The figure shows three views and two pictorial views of one solid part (mm, origin at its lowest corner). Answer the questions. A direction names the side the tool comes from. Coordinates: 2 decimals unless noted, no trailing zeros. Write each loop counter-clockwise with the first axis right and the second up, starting at its lowest first coordinate (ties: lowest second). Pieces come first, ordered by that corner, then holes.
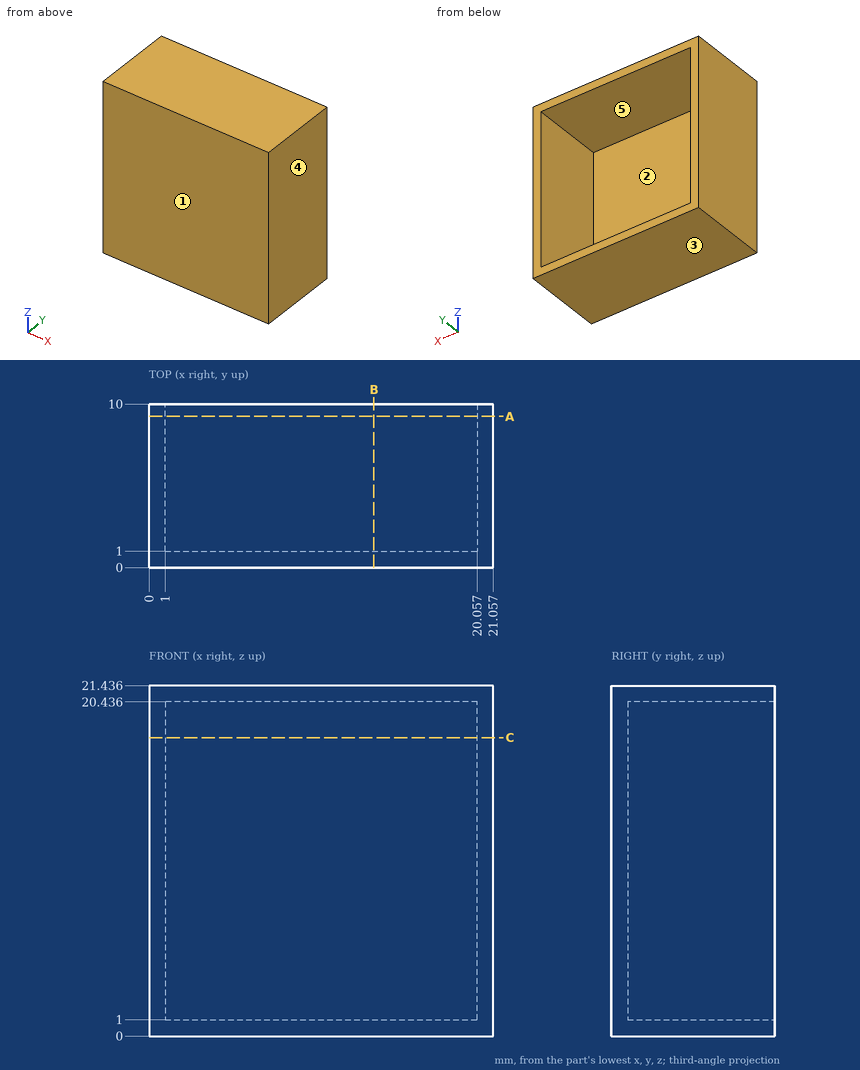
1. Section A-A on y = 9.25 is taken. Give the vertices of the cut face in (x, z) (1 decimal).
Results found:
outline: (0, 0) - (21.1, 0) - (21.1, 21.4) - (0, 21.4) - close; hole (1, 1) - (20.1, 1) - (20.1, 20.4) - (1, 20.4) - close
2. Find the intervals of material crossed by L1, parallel to X at y = 4, z = 1.25; L2, parallel to Z at x = 14, y = 7 (1 decimal); L3, parallel to Y at x = 10.5, z = 5.25, in increasing order.
Results found:
L1: x = 0 to 1, 20.06 to 21.06
L2: z = 0 to 1, 20.4 to 21.4
L3: y = 0 to 1
3. Section C-C on z = 18.25 is taken. Give the vertices of the cut face in (x, y).
Results found:
outline: (0, 0) - (21.06, 0) - (21.06, 10) - (20.06, 10) - (20.06, 1) - (1, 1) - (1, 10) - (0, 10) - close
4. Flat-ended cylindrical pins translate along their axes: P1, Ø5.5, axis at x = 13.5, z = 8, coming from the +Y side; P2, Ø4.5, axis at y = 4, z = 9.5, coming from the -X side. Find the tip coordinate at first contact, or state that the pin passes through.
Results found:
P1: stops at y = 1
P2: stops at x = 0
5. For a pull along X with two mould halves and no side action, classify the marked faces 3, 4 and 5 as pulls with the +X half, pulls with the -X half, needs draft (parallel to the pull), parting line crosses it, or undercut.
Results found:
face 3: needs draft
face 4: pulls with the +X half
face 5: undercut
6. A tool of negligible diameter and unlimited length cuts with its end or side. For the marked faces 1 and 2, from which of +Z, -Z, +X, -X, +Y, -Y can it reach the whole face along a straight path? Write none if from no direction.
Results found:
face 1: +Z, -Z, +X, -X, -Y
face 2: +Y
7. Section B-B on x = 13.75 is taken. Give the vertices of the cut face in (y, z) (1 decimal).
Results found:
outline: (0, 0) - (10, 0) - (10, 1) - (1, 1) - (1, 20.4) - (10, 20.4) - (10, 21.4) - (0, 21.4) - close
